```python
from build123d import *

# Parameters (mm, degrees)
BOSS_EXTRUDE1_DEPTH = 20
CUT_EXTRUDE2_START  = -10
CUT_EXTRUDE2_DEPTH  = 5
CUT_EXTRUDE1_START  = -36
CUT_EXTRUDE1_DEPTH  = 37
SKETCH5_W           = 3
SKETCH5_H           = 6
BOSS_EXTRUDE2_DEPTH = 2
BOSS_EXTRUDE2_TAPER = 25
FILLET1_R           = 8
CHAMFER2_SIZE       = 1
FILLET2_R           = 0.5


with BuildPart() as part:
    # Sketch1 → Boss-Extrude1 (new body)
    with BuildSketch(Plane(origin=(0, 0, 0), x_dir=(1, 0, 0), z_dir=(0, 1, 0))):
        with BuildLine():
            Line((-17.5, 15.5), (-17.5, -15.5))
            ThreePointArc((-17.5, -15.5), (-16.914213562, -16.914213562), (-15.5, -17.5))
            Line((-15.5, -17.5), (15.5, -17.5))
            ThreePointArc((15.5, -17.5), (16.914213562, -16.914213562), (17.5, -15.5))
            Line((17.5, -15.5), (17.5, -14.437438845))
            ThreePointArc((17.5, -14.437438845), (16.957737974, -13.068132452), (15.625, -12.441348918))
            ThreePointArc((15.625, -12.441348918), (-3.713203436, -3.713203436), (-12.441348918, 15.625))
            ThreePointArc((-12.441348918, 15.625), (-13.068132452, 16.957737974), (-14.437438845, 17.5))
            Line((-14.437438845, 17.5), (-15.5, 17.5))
            ThreePointArc((-15.5, 17.5), (-16.914213562, 16.914213562), (-17.5, 15.5))
        make_face()
    extrude(amount=BOSS_EXTRUDE1_DEPTH)

    # Sketch3 → Cut-Extrude2 (cut, symmetric)
    with BuildSketch(Plane(origin=(0, 20, 0), x_dir=(1, 0, 0), z_dir=(0, 1, 0)).offset(CUT_EXTRUDE2_START)):
        Polygon((-12.5, 33.240018262), (-12.5, -12.5), (41.305309001, -12.5), align=None)
    extrude(amount=CUT_EXTRUDE2_DEPTH, both=True, mode=Mode.SUBTRACT)

    # Sketch2 → Cut-Extrude1 (cut)
    with BuildSketch(Plane.ZY.offset(17.5).offset(CUT_EXTRUDE1_START)):
        with BuildLine():
            Line((-9.5, 12.75), (0.5, 12.75))
            ThreePointArc((0.5, 12.75), (3.25, 10), (0.5, 7.25))
            Line((0.5, 7.25), (-9.5, 7.25))
            ThreePointArc((-9.5, 7.25), (-12.25, 10), (-9.5, 12.75))
        make_face()
    cut_extrude1 = extrude(amount=CUT_EXTRUDE1_DEPTH, mode=Mode.SUBTRACT)

    # Sketch5 → Boss-Extrude2 (add)
    with BuildSketch(Plane.ZY.offset(17.5)):
        with Locations((-14, 10)):
            Rectangle(SKETCH5_W, SKETCH5_H)
        with Locations((14, 10)):
            Rectangle(SKETCH5_W, SKETCH5_H)
    boss_extrude2 = extrude(amount=BOSS_EXTRUDE2_DEPTH, taper=BOSS_EXTRUDE2_TAPER)

    # Mirror1: Cut-Extrude1, Boss-Extrude2 across plane
    add(cut_extrude1.mirror(Plane(origin=(0, 0, 0), x_dir=(-0.707106781, 0, 0.707106781), z_dir=(0.707106781, 0, 0.707106781))), mode=Mode.SUBTRACT)
    add(boss_extrude2.mirror(Plane(origin=(0, 0, 0), x_dir=(-0.707106781, 0, 0.707106781), z_dir=(0.707106781, 0, 0.707106781))))

    # Fillet1
    fillet1_edges = [part.edges().sort_by_distance(p)[0] for p in [
        (-12.5, 10, 12.5),
    ]]
    fillet(fillet1_edges, radius=FILLET1_R)

    # Chamfer2
    chamfer2_edges = [part.edges().sort_by_distance(p)[0] for p in [
        (-14.968719423, 0, -17.5),
        (-13.068132452, 0, -16.957737974),
        (-3.713203436, 0, 3.713203436),
        (16.957737974, 0, 13.068132452),
        (17.5, 0, 14.968719423),
        (16.914213562, 0, 16.914213562),
        (0, 0, 17.5),
        (-16.914213562, 20, 16.914213562),
        (-16.914213562, 0, 16.914213562),
        (-17.5, 0, 0),
        (-16.914213562, 0, -16.914213562),
        (0, 20, 17.5),
        (16.914213562, 20, 16.914213562),
        (17.5, 20, 14.968719423),
        (16.957737974, 20, 13.068132452),
        (-3.713203436, 20, 3.713203436),
        (-13.068132452, 20, -16.957737974),
        (-14.968719423, 20, -17.5),
        (-16.914213562, 20, -16.914213562),
        (-17.5, 20, 0),
    ]]
    chamfer(chamfer2_edges, length=CHAMFER2_SIZE)

    # Fillet2
    fillet2_edges = [part.edges().sort_by_distance(p)[0] for p in [
        (5.748158579, 5, 12.5),
        (-10.156854249, 5, 10.156854249),
        (5.748158579, 15, 12.5),
        (-10.156854249, 15, 10.156854249),
        (-12.5, 5, -5.748158579),
        (-12.5, 15, -5.748158579),
    ]]
    fillet(fillet2_edges, radius=FILLET2_R)


solid = part.part
```
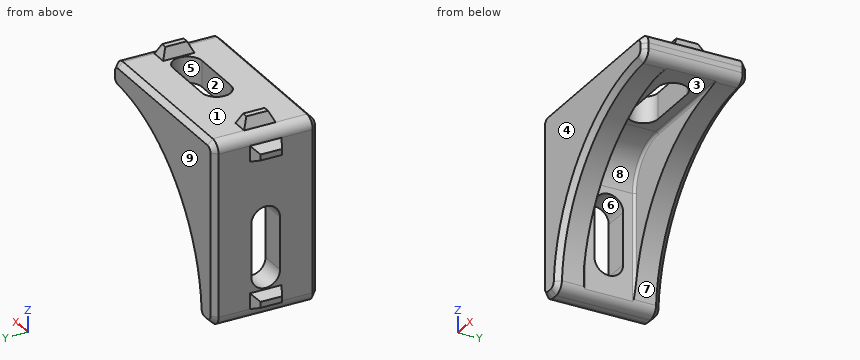
Model file for the job. Use its own axes, mm. Face numbers are marked on the shaded views. A direction names the side the tool comes from. Give positions to 0.01 mm unless a question says otherwise; leave off trailing zeros. Loops run counter-clockwise (first coordinate to the right, second up) from the corner with the lowest first, then second, coordinate; pieces in that order, holes last. Notation, with made-up numbers: (57, 29) -> (112, 29) arc R22 ccw to (112, 55) -> close; hole circle Ø6 at (-40, -3). An arc over 180 degrees is marked (long way). Write each question's results on one line, items separated by ' | '.
(1) Pull direction Y, two halves, no side cores. Call the marked faces 1, 2, 3 and 4: released by +Y, released by -Y, zero draft, split by the parting line, or undercut.
Geometry results:
face 1: zero draft | face 2: undercut | face 3: undercut | face 4: released by -Y
(2) Cut at A-A on y = 4.5. List the corners of the cut face in (x, z) (3 decimals).
Geometry results:
outline: (-17.5, -15.5) arc R2 ccw to (-15.5, -17.5) -> (-14.437, -17.5) arc R2 ccw to (-12.441, -15.625) arc R30 cw to (15.625, 12.441) arc R2 ccw to (17.5, 14.437) -> (17.5, 15.5) arc R2 ccw to (15.5, 17.5) -> (-15.5, 17.5) arc R2 ccw to (-17.5, 15.5) -> close
(3) Probe line 1 along Y through (x, z) = (-17, -7); line 2 along Z through (x, y) = (6, 14.25); line 3 along Y through (x, z) = (-10.5, -6). List the from-to ranges inside material, lowest first.
Geometry results:
line 1: y = 0.5 to 7.25, 12.75 to 19.5 | line 2: z = 12.5 to 17.5 | line 3: y = 0.73 to 5, 15 to 19.27
(4) Flat gauge pins, fed straight in: pin 1 Ø5 at (y, z) = (6.5, -6) entering from -X; pin 2 Ø19 at (x, z) = (-4, 3) entering from +Y; pin 3 Ø19 at (x, z) = (5.5, -4.5) entering from -Y; pin 4 Ø9 at (x, y) = (-5, 6.5) entering from +Z. Where does each tip first touch, or does it go through?
Geometry results:
pin 1: stops at x = -17.5 | pin 2: stops at y = 20 | pin 3: passes through | pin 4: stops at z = 17.5
(5) Cut at B-B on y = 10. Give the number of separate pieces and of enclosed holes in the cut face, and give its area (3 significant figures).
Geometry results:
separate pieces: 3 | enclosed holes: 0 | area: 196 mm²
(6) Tool access for the marked faces 5, 6, 7, 8 and 9: list every direction of +Z, -Z, +X, -X, +Y, -Y with a clear straight run to the whole face (end or side of a thin tool).
Geometry results:
face 5: +Z, -Z | face 6: +X, -X | face 7: -Z, +X, +Y, -Y | face 8: -Z, +X | face 9: +Z, -Z, +X, -X, +Y
